Input: part model. Units: mm. Frame: model coordinates. A direction names the side the tool comes from. Round coordinates to 2 decimals unless told otherwise and drop trailing zeros. Write each loop counter-clockwise with the first axis right and the second up, starting at its lowest first coordinate (ties: lowest second). Pieces come first, ordered by that corner, then holes. Notation, with made-up numbers: M 81.25,-9 L 85.25,-9 A23 ccw 85.25,0 Z; hole C 5,8.5 d2. An arc over 180 degrees is marked long. Answer as CSV lines item,"result". Start each with the question number.
```python
from build123d import *

# Parameters (mm, degrees)
F0_W     = 60
F0_H     = 40
F1_DEPTH = 10
F3_DEPTH = 2
F5_DEPTH = 4
F4_R     = 6
F6_DEPTH = 2
F2_W     = 6.3
F2_H     = 16.0467466712
F2_W_2   = 1.9639990747
F7_DEPTH = 4
F4_W     = 4.5
F4_H     = 5.2
F4_H_2   = 13
F4_W_2   = 2
F4_H_3   = 7.5
F4_R_2   = 7
F4_R_3   = 1.25
F8_DEPTH = 2


with BuildPart() as f1:
    # F0 (on Top) → F1 (new body)
    with BuildSketch(Plane.XY):
        with Locations((60.4293134809, -48.683847785)):
            Rectangle(F0_W, F0_H)
    extrude(amount=F1_DEPTH)

    # F2 (on face) → F3 (cut)
    with BuildSketch(Plane.XY.offset(10)):
        with BuildLine():
            Line((38.4793134809, -32.283847785), (36.7293134809, -32.283847785))
            Line((36.7293134809, -32.283847785), (36.7293134809, -34.033847785))
            ThreePointArc((36.7293134809, -34.033847785), (37.9667503479, -33.5212846521), (38.4793134809, -32.283847785))
        make_face()
        with BuildLine():
            Line((36.7293134809, -34.033847785), (36.7293134809, -32.283847785))
            Line((36.7293134809, -32.283847785), (38.4793134809, -32.283847785))
            ThreePointArc((38.4793134809, -32.283847785), (35.4918766138, -31.0464109179), (36.7293134809, -34.033847785))
        make_face()
        with BuildLine():
            ThreePointArc((38.4793134809, -65.083847785), (37.9667503479, -63.8464109179), (36.7293134809, -63.333847785))
            Line((36.7293134809, -63.333847785), (36.7293134809, -65.083847785))
            Line((36.7293134809, -65.083847785), (38.4793134809, -65.083847785))
        make_face()
        with BuildLine():
            Line((36.7293134809, -65.083847785), (36.7293134809, -63.333847785))
            ThreePointArc((36.7293134809, -63.333847785), (35.4918766138, -66.3212846521), (38.4793134809, -65.083847785))
            Line((38.4793134809, -65.083847785), (36.7293134809, -65.083847785))
        make_face()
        with BuildLine():
            ThreePointArc((85.8793134809, -65.083847785), (85.3667503479, -63.8464109179), (84.1293134809, -63.333847785))
            Line((84.1293134809, -63.333847785), (84.1293134809, -65.083847785))
            Line((84.1293134809, -65.083847785), (82.3793134809, -65.083847785))
            ThreePointArc((82.3793134809, -65.083847785), (84.1293134809, -66.833847785), (85.8793134809, -65.083847785))
        make_face()
        with BuildLine():
            Line((84.1293134809, -65.083847785), (84.1293134809, -63.333847785))
            ThreePointArc((84.1293134809, -63.333847785), (82.8918766138, -63.8464109179), (82.3793134809, -65.083847785))
            Line((82.3793134809, -65.083847785), (84.1293134809, -65.083847785))
        make_face()
        with BuildLine():
            Line((82.3793134809, -32.283847785), (38.4793134809, -32.283847785))
            ThreePointArc((38.4793134809, -32.283847785), (37.9667503479, -33.5212846521), (36.7293134809, -34.033847785))
            Line((36.7293134809, -34.033847785), (36.7293134809, -40.6604744494))
            Line((36.7293134809, -40.6604744494), (38.6933125556, -40.6604744494))
            Line((38.6933125556, -40.6604744494), (38.6933125556, -56.7072211206))
            Line((38.6933125556, -56.7072211206), (36.7293134809, -56.7072211206))
            Line((36.7293134809, -56.7072211206), (36.7293134809, -63.333847785))
            ThreePointArc((36.7293134809, -63.333847785), (37.9667503479, -63.8464109179), (38.4793134809, -65.083847785))
            Line((38.4793134809, -65.083847785), (82.3793134809, -65.083847785))
            ThreePointArc((82.3793134809, -65.083847785), (82.8918766138, -63.8464109179), (84.1293134809, -63.333847785))
            Line((84.1293134809, -63.333847785), (84.1293134809, -34.033847785))
            ThreePointArc((84.1293134809, -34.033847785), (82.8918766138, -33.5212846521), (82.3793134809, -32.283847785))
        make_face()
        with BuildLine():
            Line((84.1293134809, -32.283847785), (82.3793134809, -32.283847785))
            ThreePointArc((82.3793134809, -32.283847785), (82.8918766138, -33.5212846521), (84.1293134809, -34.033847785))
            Line((84.1293134809, -34.033847785), (84.1293134809, -32.283847785))
        make_face()
        with BuildLine():
            ThreePointArc((85.8793134809, -32.283847785), (84.1293134809, -30.533847785), (82.3793134809, -32.283847785))
            Line((82.3793134809, -32.283847785), (84.1293134809, -32.283847785))
            Line((84.1293134809, -32.283847785), (84.1293134809, -34.033847785))
            ThreePointArc((84.1293134809, -34.033847785), (85.3667503479, -33.5212846521), (85.8793134809, -32.283847785))
        make_face()
    extrude(amount=-F3_DEPTH, mode=Mode.SUBTRACT)

    # F2 (on face) → F5 (cut)
    with BuildSketch(Plane.XY.offset(10)):
        with BuildLine():
            Line((38.4793134809, -32.283847785), (36.7293134809, -32.283847785))
            Line((36.7293134809, -32.283847785), (36.7293134809, -34.033847785))
            ThreePointArc((36.7293134809, -34.033847785), (37.9667503479, -33.5212846521), (38.4793134809, -32.283847785))
        make_face()
        with BuildLine():
            Line((36.7293134809, -34.033847785), (36.7293134809, -32.283847785))
            Line((36.7293134809, -32.283847785), (38.4793134809, -32.283847785))
            ThreePointArc((38.4793134809, -32.283847785), (35.4918766138, -31.0464109179), (36.7293134809, -34.033847785))
        make_face()
        with BuildLine():
            ThreePointArc((38.4793134809, -65.083847785), (37.9667503479, -63.8464109179), (36.7293134809, -63.333847785))
            Line((36.7293134809, -63.333847785), (36.7293134809, -65.083847785))
            Line((36.7293134809, -65.083847785), (38.4793134809, -65.083847785))
        make_face()
        with BuildLine():
            Line((36.7293134809, -65.083847785), (36.7293134809, -63.333847785))
            ThreePointArc((36.7293134809, -63.333847785), (35.4918766138, -66.3212846521), (38.4793134809, -65.083847785))
            Line((38.4793134809, -65.083847785), (36.7293134809, -65.083847785))
        make_face()
        with BuildLine():
            Line((84.1293134809, -32.283847785), (82.3793134809, -32.283847785))
            ThreePointArc((82.3793134809, -32.283847785), (82.8918766138, -33.5212846521), (84.1293134809, -34.033847785))
            Line((84.1293134809, -34.033847785), (84.1293134809, -32.283847785))
        make_face()
        with BuildLine():
            ThreePointArc((85.8793134809, -32.283847785), (84.1293134809, -30.533847785), (82.3793134809, -32.283847785))
            Line((82.3793134809, -32.283847785), (84.1293134809, -32.283847785))
            Line((84.1293134809, -32.283847785), (84.1293134809, -34.033847785))
            ThreePointArc((84.1293134809, -34.033847785), (85.3667503479, -33.5212846521), (85.8793134809, -32.283847785))
        make_face()
        with BuildLine():
            Line((84.1293134809, -65.083847785), (84.1293134809, -63.333847785))
            ThreePointArc((84.1293134809, -63.333847785), (82.8918766138, -63.8464109179), (82.3793134809, -65.083847785))
            Line((82.3793134809, -65.083847785), (84.1293134809, -65.083847785))
        make_face()
        with BuildLine():
            ThreePointArc((85.8793134809, -65.083847785), (85.3667503479, -63.8464109179), (84.1293134809, -63.333847785))
            Line((84.1293134809, -63.333847785), (84.1293134809, -65.083847785))
            Line((84.1293134809, -65.083847785), (82.3793134809, -65.083847785))
            ThreePointArc((82.3793134809, -65.083847785), (84.1293134809, -66.833847785), (85.8793134809, -65.083847785))
        make_face()
    extrude(amount=-F5_DEPTH, mode=Mode.SUBTRACT)

    # F4 (on face) → F6 (join)
    with BuildSketch(Plane.XY.offset(8)):
        with Locations((71.2293134809, -46.683847785)):
            Circle(F4_R)
    extrude(amount=F6_DEPTH)

    # F2 (on face) → F7 (cut)
    with BuildSketch(Plane.XY.offset(10)):
        with Locations((33.5793134809, -48.683847785)):
            Rectangle(F2_W, F2_H)
        with Locations((37.7113130182, -48.683847785)):
            Rectangle(F2_W_2, F2_H)
    extrude(amount=-F7_DEPTH, mode=Mode.SUBTRACT)

    # F4 (on face) → F8 (cut)
    with BuildSketch(Plane.XY.offset(8)):
        with BuildLine():
            Line((78.1293134809, -33.283847785), (42.7293134809, -33.283847785))
            ThreePointArc((42.7293134809, -33.283847785), (39.1937795749, -34.7483138791), (37.7293134809, -38.283847785))
            Line((37.7293134809, -38.283847785), (37.7293134809, -40.6604744494))
            Line((37.7293134809, -40.6604744494), (38.6933125556, -40.6604744494))
            Line((38.6933125556, -40.6604744494), (38.6933125556, -56.7072211206))
            Line((38.6933125556, -56.7072211206), (37.7293134809, -56.7072211206))
            Line((37.7293134809, -56.7072211206), (37.7293134809, -59.028696239))
            ThreePointArc((37.7293134809, -59.028696239), (39.1937795749, -62.5642301449), (42.7293134809, -64.028696239))
            Line((42.7293134809, -64.028696239), (44.9293134809, -64.028696239))
            ThreePointArc((44.9293134809, -64.028696239), (47.0506338244, -63.1500165826), (47.9293134809, -61.028696239))
            Line((47.9293134809, -61.028696239), (47.9293134809, -58.828696239))
            Line((47.9293134809, -58.828696239), (52.4293134809, -58.828696239))
            Line((52.4293134809, -58.828696239), (52.4293134809, -61.028696239))
            ThreePointArc((52.4293134809, -61.028696239), (53.3079931373, -63.1500165826), (55.4293134809, -64.028696239))
            Line((55.4293134809, -64.028696239), (66.2293134809, -64.028696239))
            ThreePointArc((66.2293134809, -64.028696239), (68.3506338244, -63.1500165826), (69.2293134809, -61.028696239))
            Line((69.2293134809, -61.028696239), (69.2293134809, -60.028696239))
            Line((69.2293134809, -60.028696239), (80.1293134809, -60.028696239))
            ThreePointArc((80.1293134809, -60.028696239), (82.2506338244, -59.1500165826), (83.1293134809, -57.028696239))
            Line((83.1293134809, -57.028696239), (83.1293134809, -38.283847785))
            ThreePointArc((83.1293134809, -38.283847785), (81.6648473868, -34.7483138791), (78.1293134809, -33.283847785))
        make_face()
        with Locations((50.1793134809, -49.883847785)):
            Rectangle(F4_W, F4_H, mode=Mode.SUBTRACT)
        with Locations((56.9793134809, -51.783847785)):
            Rectangle(F4_W, F4_H_2, mode=Mode.SUBTRACT)
        with Locations((44.7293134809, -48.533847785)):
            Rectangle(F4_W_2, F4_H_3, mode=Mode.SUBTRACT)
        with Locations((71.2293134809, -46.683847785)):
            Circle(F4_R_2, mode=Mode.SUBTRACT)
        with Locations((79.6293134809, -37.583847785)):
            Circle(F4_R_3, mode=Mode.SUBTRACT)
    extrude(amount=-F8_DEPTH, mode=Mode.SUBTRACT)


solid = f1.part
```
Item 1: Cut plane B-B, the plane y = -46. Return loops of the section in (x, z).
Item 2: Cut plane C-C, the plane y = -35.5. Return loops of the section in (x, z), plus the area to 3 significant figures.
Item 3: Draft query along Y for faces 3 (the face through (35.34, -66.15, 8.03)), 4 (the face through (56, -45, 6)), 5 (the face through (60, -68.684, 5)). Return one class per face: +Y half, -Y half, draft (parallel to the pull), parting line (faces both ways), or undercut.
Item 4: Cut plane A-A, the plane x = 50. Return loops of the section in (y, z).
Item 5: Line query: line 1 (Y direction, x = 57.5, z = 6.25); line 2 (Y direction, x = 70, z = 8.5); line 3 (X direction, y = -66, z = 7). Output: solid intervals per line, ascending. Write a range as [from, to].
Item 6: Access query for faces 1 (the face through (37.729, -39, 7)), 2 (the face through (43.729, -49, 7)). Directions: +Z, -Z, +X, -X, +Y, -Y. A direction counts if a zero-diameter tool reaches every point of the face in a straight line with its end or side. Return the directions, or none.
Item 7: Cut plane D-D, the plane x = 73. Return loops of the section in (y, z).
Item 8: Pin query (flat end, axial travel): pin 1 Ø0.8 at (x, y) = (80, -37.5) entering from +Z; pin 2 Ø0.6 at (y, z) = (-50, 7) entering from -X; pin 3 Ø2 at (y, z) = (-55, 7.5) entering from -X. Return the tip coordinate at first contact, or that it passes through.
Results list:
1,outline,"M 30.43,0 L 90.43,0 L 90.43,10 L 84.13,10 L 84.13,8 L 83.13,8 L 83.13,6 L 78.2,6 L 78.2,8 L 77.19,8 L 77.19,10 L 65.27,10 L 65.27,8 L 64.26,8 L 64.26,6 L 59.23,6 L 59.23,8 L 54.73,8 L 54.73,6 L 45.73,6 L 45.73,8 L 43.73,8 L 43.73,6 L 30.43,6 Z"
2,outline,"M 30.43,0 L 90.43,0 L 90.43,10 L 84.13,10 L 84.13,8 L 82.28,8 L 82.28,6 L 38.58,6 L 38.58,8 L 36.73,8 L 36.73,10 L 30.43,10 Z"
2,area,"418 mm²"
3,face 3,"undercut"
3,face 4,"undercut"
3,face 5,"-Y half"
4,outline,"M -68.68,0 L -28.68,0 L -28.68,10 L -32.28,10 L -32.28,8 L -33.28,8 L -33.28,6 L -47.28,6 L -47.28,8 L -52.48,8 L -52.48,6 L -58.83,6 L -58.83,8 L -65.08,8 L -65.08,10 L -68.68,10 Z"
5,line 1,"[-68.68, -64.03], [-58.28, -45.28], [-33.28, -28.68]"
5,line 2,"[-68.68, -65.08], [-52.56, -40.81], [-32.28, -28.68]"
5,line 3,"[30.43, 35.24], [38.22, 82.64], [85.62, 90.43]"
6,face 1,"+Z"
6,face 2,"+Z, -X"
7,outline,"M -68.68,0 L -28.68,0 L -28.68,10 L -32.28,10 L -32.28,8 L -33.28,8 L -33.28,6 L -39.91,6 L -39.91,8 L -40.95,8 L -40.95,10 L -52.42,10 L -52.42,8 L -53.46,8 L -53.46,6 L -60.03,6 L -60.03,8 L -65.08,8 L -65.08,10 L -68.68,10 Z"
8,pin 1,"z = 8"
8,pin 2,"x = 43.73"
8,pin 3,"x = 54.73"
